The listing builds one solid part. Answer for the finished solid, in the listing's coordinates (mm). A direction names the side the tool comes from. Give positions to 0.01 mm unless a question says otherwise; leave off trailing zeros. Write each loop counter-clockwise with the first axis right and the second up, starting at its lowest first coordinate (ties: lowest second). Pieces come first, ordered by that corner, then holes. Notation, with made-up numbers: (-28, -2) - (-14, -2) arc R7 cw to (-14, 8) - close; hole circle Ø2 at (29.5, 11). An arc over 180 degrees is marked (long way). Return JSON: item names as keys, results as strings.
from build123d import *

# Parameters (mm, degrees)
SKETCH_1_W          = 41
SKETCH_1_H          = 41
EXTRUDE_1_DEPTH     = 41
SKETCH_2_R          = 15
CUT_EXTRUDE_1_DEPTH = 5
FILLET_1_R          = 5


with BuildPart() as part:
    # 草图1 → 凸台-拉伸1 (new body)
    with BuildSketch(Plane.XY):
        Rectangle(SKETCH_1_W, SKETCH_1_H)
    extrude(amount=EXTRUDE_1_DEPTH)

    # 草图2 → 切除-拉伸1 (cut)
    with BuildSketch(Plane.XY.offset(41)):
        Circle(SKETCH_2_R)
    extrude(amount=-CUT_EXTRUDE_1_DEPTH, mode=Mode.SUBTRACT)

    # 圆角1
    fillet_1_edges = [part.edges().sort_by_distance(p)[0] for p in [
        (20.5, -20.5, 20.5),
        (-20.5, -20.5, 20.5),
        (-20.5, 20.5, 20.5),
        (20.5, 20.5, 20.5),
    ]]
    fillet(fillet_1_edges, radius=FILLET_1_R)


solid = part.part
Item 1: A cutting plane is placed at A-A on x = 0. Determine the outline of the cut face in (y, z).
Answer below:
{"outline": "(-20.5, 0) - (20.5, 0) - (20.5, 41) - (15, 41) - (15, 36) - (-15, 36) - (-15, 41) - (-20.5, 41) - close"}
Item 2: The mould has two halves that part along Y. Classify faces 1 (the face through (19, -19.07, 20.79)), 2 (the face through (0, 0, 36)), 3 (the face through (-19.07, 19, 20.79)): +Y half, -Y half, draft (parallel to the pull), parting line (faces both ways), or undercut.
Answer below:
{"face 1": "-Y half", "face 2": "undercut", "face 3": "+Y half"}
Item 3: A cutting plane is placed at C-C on x = -18. Determine the outline of the cut face in (y, z).
Answer below:
{"outline": "(-19.83, 0) - (19.83, 0) - (19.83, 41) - (-19.83, 41) - close"}
Item 4: A flat-ended cylindrical pin translates along its axis: P1, Ø3, axis at x = -2.5, y = -10.5, coming from the +Z side. Find the tip coordinate at first contact, or state that the pin passes through.
Answer below:
{"P1": "stops at z = 36"}
Item 5: Consider L1, parallel to Y at x = 0, z = 39.75; L2, parallel to Z at x = -0.5, y = -9.5; L3, parallel to Y at x = 12.5, z = 39.5. Determine where each line is inside the solid, lowest interval first.
Answer below:
{"L1": "y = -20.5 to -15, 15 to 20.5", "L2": "z = 0 to 36", "L3": "y = -20.5 to -8.29, 8.29 to 20.5"}
Item 6: For faces 4 (the face through (0, 0, 0)), 5 (the face through (-14.985, 0.66, 38.535)), determine the directions among +Z, -Z, +X, -X, +Y, -Y from which every point of the face is accessible in a straight line to the end or side of a thin tool.
Answer below:
{"face 4": "-Z, +X, -X, +Y, -Y", "face 5": "+Z"}
